```python
from build123d import *

# Parameters (mm, degrees)
SKETCH3_R                = 9.525
BOSS_EXTRUDE1_DEPTH      = 2.38125
BOSS_EXTRUDE4_DEPTH      = 25.4
SKETCH7_W                = 5.08
SKETCH7_H                = 1.016
BOSS_EXTRUDE5_DEPTH      = 12.7
CUT_EXTRUDE1_DEPTH       = 1.27
BOSS_EXTRUDE6_DEPTH      = 0.508
BOSS_EXTRUDE6_DEPTH_BACK = 9.398
SKETCH11_R               = 2.54
BOSS_EXTRUDE7_DEPTH      = 24.13


with BuildPart() as part:
    # Sketch3 → Boss-Extrude1 (new, symmetric)
    with BuildSketch(Plane(origin=(0, 0, 0), x_dir=(0, 1, 0), z_dir=(0, 0, 1))):
        with Locations(Location((0, 0, 0), (0, 0, 90))):
            Circle(SKETCH3_R)
    extrude(amount=BOSS_EXTRUDE1_DEPTH, both=True)



with BuildPart() as body_2:
    # Sketch6 → Boss-Extrude4 (new body)
    with BuildSketch(Plane.YZ.offset(9.525)):
        Polygon((-5.08, 0), (-2.54, -4.399409051), (2.54, -4.399409051), (5.08, 0), (2.54, 4.399409051), (-2.54, 4.399409051), align=None)
    extrude(amount=BOSS_EXTRUDE4_DEPTH)

    # Sketch7 → Boss-Extrude5 (add)
    with BuildSketch(Plane(origin=(9.525, 0, 0), x_dir=(0, -1, 0), z_dir=(-1, 0, 0))):
        with Locations((0, 3.891409051)):
            Rectangle(SKETCH7_W, SKETCH7_H)
        with Locations((0, -3.891409051)):
            Rectangle(SKETCH7_W, SKETCH7_H)
    extrude(amount=BOSS_EXTRUDE5_DEPTH)

    # Sketch10 → Cut-Extrude1 (cut)
    with BuildSketch(Plane(origin=(9.525, 0, 0), x_dir=(0, -1, 0), z_dir=(-1, 0, 0))):
        Polygon((-2.54, 4.399409051), (-5.08, 0), (-2.54, -4.399409051), (-2.54, -3.383409051), (2.54, -3.383409051), (2.54, -4.399409051), (5.08, 0), (2.54, 4.399409051), (2.54, 3.383409051), (-2.54, 3.383409051), align=None)
    extrude(amount=-CUT_EXTRUDE1_DEPTH, mode=Mode.SUBTRACT)


with BuildPart() as part_1:
    add(part.part)

    add(body_2.part)  # Boss-Extrude6 merges body 2
    # Sketch11 → Boss-Extrude6 (add, two sides: drawn at the far end of the back side and taken through both)
    with BuildSketch(Plane.XY.offset(4.399409051).offset(-BOSS_EXTRUDE6_DEPTH_BACK)):
        Circle(SKETCH11_R)
    extrude(amount=BOSS_EXTRUDE6_DEPTH + BOSS_EXTRUDE6_DEPTH_BACK)

    # Sketch12 → Boss-Extrude7 (add)
    with BuildSketch(Plane.YZ.offset(34.925)):
        Polygon((-10.16, 0), (-5.08, -8.798818102), (5.08, -8.798818102), (10.16, 0), (5.08, 8.798818102), (-5.08, 8.798818102), align=None)
    extrude(amount=-BOSS_EXTRUDE7_DEPTH)


solid = part_1.part
```
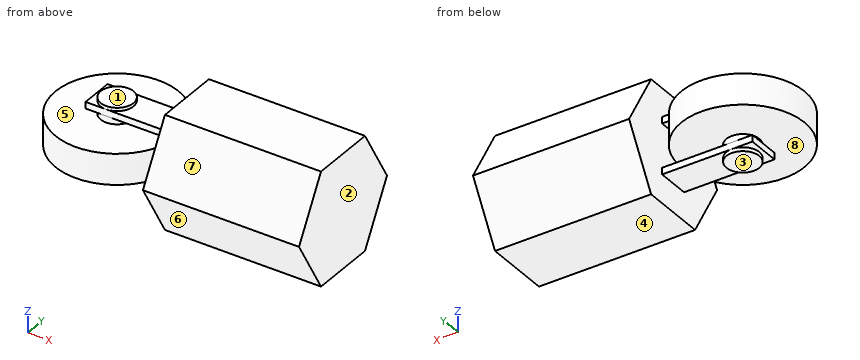
Check sheet for the modelled part. Datum: model origin and axes. Units: mm. Face numbers are marked on the shaded views. A direction names the side the tool comes from. Coordinates: 2 decimals unless noted, no trailing zeros. Loops run counter-clockwise (first coordinate to the right, second up) from the corner with the lowest first, then second, coordinate; pieces in that order, holes last. Notation, with made-up numbers: M 17,19 L 61,19 A28 ccw 61,40 Z; hole C -10,-36.75 d8. An arc over 180 degrees is marked long. Answer as a JSON object with one key per item and string values.
1. Release check for a two-part mould opening along Z. For the marked faces 6, 7 and 8 record: pulls with the +Z half, pulls with the -Z half, needs draft (parallel to the pull), parting line crosses it, or undercut.
Outcome:
{"face 6": "pulls with the -Z half", "face 7": "pulls with the +Z half", "face 8": "undercut"}
2. Sectioned sample at D-D on x = 6.5. Record the cut outline in (y, z).
Outcome:
{"outline": "M -6.96,-2.38 L 6.96,-2.38 L 6.96,2.38 L -6.96,2.38 Z; M -2.54,-4.4 L 2.54,-4.4 L 2.54,-3.38 L -2.54,-3.38 Z; M -2.54,3.38 L 2.54,3.38 L 2.54,4.4 L -2.54,4.4 Z"}
3. Depth check by flat-ended pin: P1, Ø0.5, axis at y = 0.5, z = -4, coming from the -X side (3 decimals); P2, Ø3, axis at x = 7, z = 0.5, coming from the -Y side; P3, Ø1.6, axis at x = -2, y = -1, coming from the -Z side. Enter the tip coordinate at first touch or a pass-through.
Outcome:
{"P1": "x = -3.175", "P2": "y = -7.78", "P3": "z = -5"}
4. Sectioned sample at B-B on z = -1. Record the cut outline in (x, y) (3 decimals), and give its area (3 significant figures).
Outcome:
{"outline": "C 0,0 d19.05; M 10.795,-9.583 L 34.925,-9.583 L 34.925,9.583 L 10.795,9.583 Z", "area": "747 mm²"}
5. Access from +Z, -Z, +X, -X, +Y, -Y to the whole of each face (thin tool, end or side, straight path). Record for the marked faces 1, 2, 3, 4 and 5.
Outcome:
{"face 1": "+Z, -X, +Y, -Y", "face 2": "+Z, -Z, +X, +Y, -Y", "face 3": "-Z, -X, +Y, -Y", "face 4": "-Z, +X, -X, +Y, -Y", "face 5": "none"}
6. Sectioned sample at C-C on y = 7.5. Record the cut outline in (x, z) (3 decimals).
Outcome:
{"outline": "M -5.872,-2.381 L 5.872,-2.381 L 5.872,2.381 L -5.872,2.381 Z; M 10.795,-4.607 L 34.925,-4.607 L 34.925,4.607 L 10.795,4.607 Z"}
7. Scan lines: L1, parallel to Y at x = 3, z = -4; L2, parallel to Z at x = 2.5, y = -4.25; L3, parallel to X at y = -4.5, z = 7 (3 decimals). Record each from-to range of solid material in increasing order. Write a range as from..to.
Outcome:
{"L1": "-2.54..2.54", "L2": "-2.38..2.38", "L3": "10.795..34.925"}
